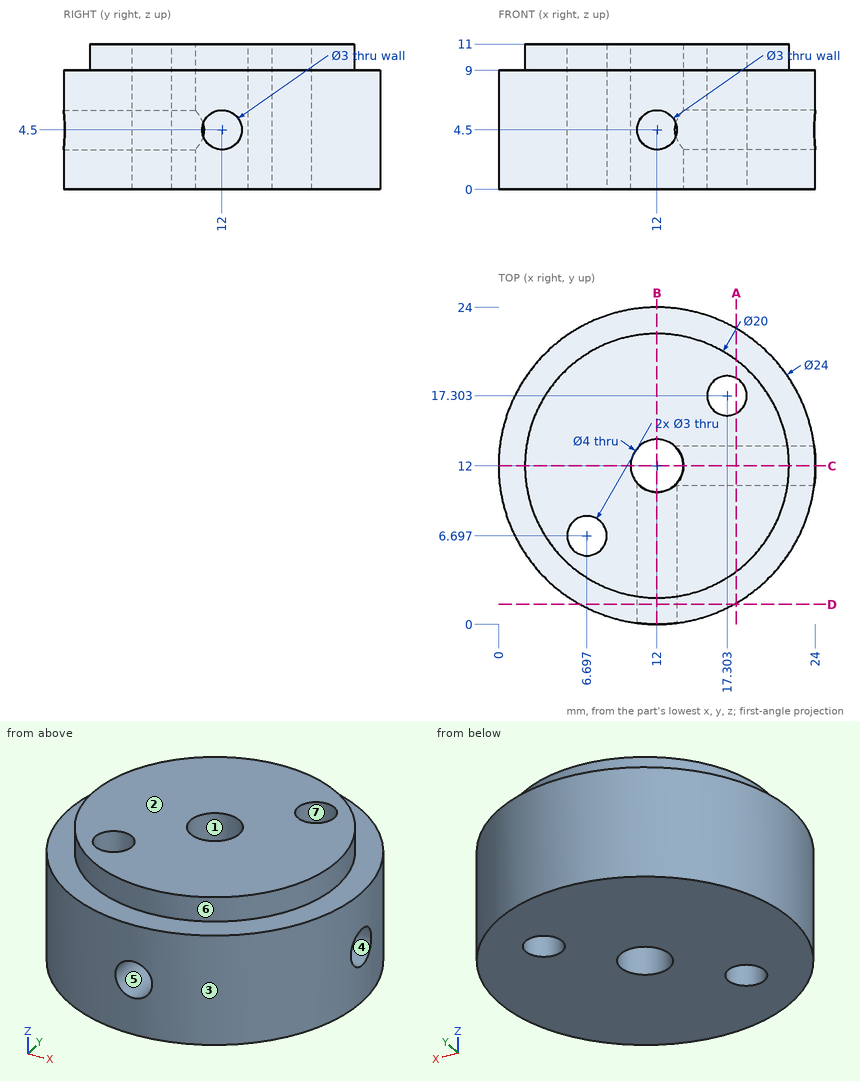
Print and shaded views of the part. All mm, measured from the part's lowest x, y and z. A direction names the side the tool comes from. Coordinates: 2 decimals unless noted, no trailing zeros. Order: outer loops, then holes, each group sorted by start corner. A loop starts at its lowest first (then second) coordinate and runs counter-clockwise, first axis right, second up. Notation, with made-up numbers: (62.5, -32.5) - (119.5, -32.5) arc R5 cw to (119.5, -23.5) - close; hole circle Ø8 at (13, -0.75). An arc over 180 degrees is marked (long way). Put each result on its own line as item: value.
1. Pull direction Y, two halves, no side cores. Call the marked faces 1, 2, 3 and 4: pulls with the +Y half, pulls with the -Y half, needs draft (parallel to the pull), parting line crosses it, or undercut.
Answer sheet:
face 1: undercut
face 2: needs draft
face 3: parting line crosses it
face 4: undercut
2. Saw through at B-B (x = 12). Write the cut outline in (y, z).
Answer sheet:
outline: (0, 0) - (10, 0) - (10, 3) - (0, 3) - close; (0, 6) - (10, 6) - (10, 11) - (2, 11) - (2, 9) - (0, 9) - close; (14, 0) - (24, 0) - (24, 9) - (22, 9) - (22, 11) - (14, 11) - close
3. Saw through at C-C (y = 12). Write the cut outline in (x, z), and give its area (3 significant figures).
Answer sheet:
outline: (0, 0) - (10, 0) - (10, 11) - (2, 11) - (2, 9) - (0, 9) - close; (14, 0) - (24, 0) - (24, 3) - (14, 3) - close; (14, 6) - (24, 6) - (24, 9) - (22, 9) - (22, 11) - (14, 11) - close
area: 182 mm^2
4. Saw through at A-A (x = 18). Write the cut outline in (y, z) (1 decimal), and give its area (3 significant figures).
Answer sheet:
outline: (1.6, 0) - (16, 0) - (16, 11) - (4, 11) - (4, 9) - (1.6, 9) - close; (18.6, 0) - (22.4, 0) - (22.4, 9) - (20, 9) - (20, 11) - (18.6, 11) - close; hole circle Ø3 at (12, 4.5)
area: 183 mm^2
5. Saw through at D-D (y = 1.5). Write the cut outline in (x, z).
Answer sheet:
outline: (6.19, 0) - (17.81, 0) - (17.81, 9) - (6.19, 9) - close; hole circle Ø3 at (12, 4.5)
6. Probe line 1 along Y through (x, z) = (12, 2.75); line 2 along Y through (x, z) = (16.5, 3.25) (1 decimal); line 3 along Z through (x, y) = (16.75, 1.75). List the from-to ranges inside material, lowest first. Write a range as [from, to].
Answer sheet:
line 1: y = [0, 10], [14, 24]
line 2: y = [0.9, 11.2], [12.8, 16], [18.6, 23.1]
line 3: z = [0, 9]
7. Tool access for the marked faces 5, 6 and 7: list every direction of +Z, -Z, +X, -X, +Y, -Y with a clear straight run to the whole face (end or side of a thin tool).
Answer sheet:
face 5: -Y
face 6: +Z
face 7: +Z, -Z
8. Drop flat-ended pins along their axis: P1, Ø1, axis at x = 11, z = 3.5, coming from the -Y side; P2, Ø1.5, axis at x = 20, y = 21, coming from the +Z side; P3, Ø2.5, axis at x = 12, z = 4.5, coming from the -Y side; P4, Ø2.5, axis at x = 6.7, y = 6.7, coming from the -Z side. Give the stop position or say it passes through.
Answer sheet:
P1: stops at y = 0.02
P2: stops at z = 9
P3: stops at y = 13.56
P4: passes through
